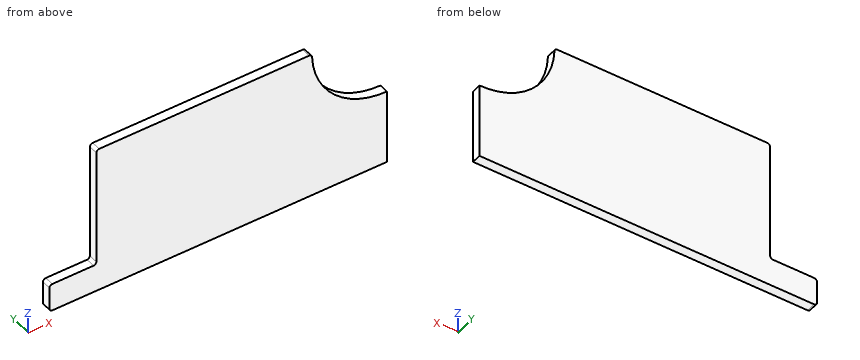
Autodesk Inventor part; units mm, degrees
ref_plane "YZ Plane" through (0, 0, 0) normal (1, 0, 0) x (0, 1, 0)
ref_plane "XZ Plane" through (0, 0, 0) normal (0, 1, 0) x (-1, 0, 0)
ref_plane "XY Plane" through (0, 0, 0) normal (0, 0, 1) x (1, 0, 0)
sketch "Esboço1" plane through (0, 0, 0) normal (0, 1, 0) x (-1, 0, 0)
  line L0 (-900, 400) -> (900, 400) construction
  line L1 (900, 400) -> (900, -400) construction
  line L2 (900, -400) -> (-900, -400) construction
  line L3 (-900, -400) -> (-900, 400) construction
  line L4 (-900, 400) -> (900, -400) construction
  line L5 (900, 400) -> (-900, -400) construction
  line L6 (900, -250) -> (650, -250) construction
  line L7 (650, -250) -> (650, 400) construction
  arc A0 (885, -400) -> (900, -385) centre (885, -385) ccw
  arc A1 (650, -235) -> (665, -250) centre (665, -235) ccw
  line L8 (885, -400) -> (-900, -400)
  line L9 (900, -385) -> (900, -250) construction
  line L10 (900, -250) -> (665, -250) construction
  line L11 (-900, -400) -> (-1700, -400) construction
  line L12 (-1700, -400) -> (-1700, 1400) construction
  line L13 (-1700, 1400) -> (-900, 1400) construction
  line L14 (-900, 1400) -> (-900, -400) construction
  circle A2 centre (-900, 400) radius 400 construction
  line L15 (900, 0) -> (-900, 0) construction
  line L16 (-1300, 1400) -> (-1300, -404.7673) construction
  arc A3 (-485.2712, 400) -> (-500.2614, 385.5422) centre (-485.2712, 385) ccw
  line L17 (650, -235) -> (650, 385)
  arc A4 (650, 385) -> (635, 400) centre (635, 385) ccw
  line L18 (635, 400) -> (-485.2712, 400)
  arc A5 (-900, 0) -> (-500.2614, 385.5422) centre (-900, 400) ccw
  line L19 (-900, -400) -> (-900, 0)
  arc A6 (900, -265) -> (885, -250) centre (885, -265) ccw
  line L20 (900, -265) -> (900, -385)
  line L21 (885, -250) -> (665, -250)
  point P0 (0, 0)
  dimension "d11" = 800
  dimension "d0" = 800
  dimension "d1" = 1800
  dimension "d3" = 650
  dimension "d5" = 15
  dimension "d6" = 800
  dimension "d7" = 1800
  dimension "d9" = 250
  dimension "d13" = 400
  dimension "d14" = 400
  dimension "d15" = 400
sketch "Esboço3" plane through (0, 0, 0) normal (0, 1, 0) x (-1, 0, 0)
  line L0 (-900, 400) -> (900, 400) construction
  line L1 (900, 400) -> (900, -400) construction
  line L2 (900, -400) -> (-900, -400) construction
  line L3 (-900, -400) -> (-900, 400) construction
  line L4 (-900, 400) -> (900, -400) construction
  line L5 (900, 400) -> (-900, -400) construction
  arc A0 (-900, -350) -> (-850, -400) centre (-850, -350) ccw
  arc A1 (850, -400) -> (900, -350) centre (850, -350) ccw
  line L6 (900, 0) -> (-900, 0) construction
  line L7 (700, 400) -> (700, 0) construction
  line L8 (850, -400) -> (-850, -400)
  line L9 (900, -350) -> (900, 400)
  line L10 (-900, -350) -> (-900, -350)
  line L11 (-900, -309.491) -> (-900, -350)
  arc A2 (-850, 400) -> (-900, 350) centre (-850, 350) ccw
  line L12 (-900, -309.491) -> (-900, 350)
  circle A3 centre (300, 400) radius 400 construction
  arc A4 (-97.5232, 355.5556) -> (-147.2136, 400) centre (-147.2136, 350) ccw
  line L13 (900, 400) -> (700, 400)
  line L14 (-147.2136, 400) -> (-850, 400)
  arc A5 (-97.5232, 355.5556) -> (700, 400) centre (300, 400) ccw
  point P0 (0, 0)
  point P1 (-498.6068, 400)
  dimension "d16" = 1800
  dimension "d17" = 800
  dimension "d19" = 200
  dimension "d20" = 50
  dimension "d21" = 800
extrude "Extrusão1" add sketch "Esboço1" along normal mid plane 50
equation "\"d6\" = d0"
equation "\"d7\" = d1"
properties part number "Lado Esquerdo Mesa"
Work out the finished part from the listing and answer in its coordinate system (mm). Give positions to 0.01 mm unless a question says otherwise; leave off trailing zeros. Order: outer loops, then holes, each group sorted by start corner. A loop starts at its lowest first (then second) coordinate and runs counter-clockwise, first axis right, second up. Notation, with made-up numbers: M 61.5,20 L 72.5,20 A26 ccw 72.5,34 Z; hole C -17,57.25 d1. An arc over 180 degrees is marked long. Return JSON: item names as keys, results as strings.
1) Section C-C, the plane x = -705 is taken. Write down the section's boundary in (y, z), plus the area to 3 significant figures.
Resolved:
{"outline": "M -25,-400 L 25,-400 L 25,-250 L -25,-250 Z", "area": "7,500 mm^2"}
2) Each of these flat-tipped pins is pushed along its axis until it touches: pin 1 (2 mm diameter, centred on y = 4, z = 311.5, fed in from -X); pin 2 (6 mm diameter, centred on y = 7, z = 231, fed in from +X). Where does it stop, or does it pass through?
Resolved:
{"pin 1": "x = -650", "pin 2": "x = 538.87"}
3) Section A-A, the plane y = -16 is taken. Write down the section's boundary in (x, z), plus the area to 3 significant figures.
Resolved:
{"outline": "M -900,-385 A15 ccw -885,-400 L 900,-400 L 900,0 A400 cw 500.26,385.54 A15 ccw 485.27,400 L -635,400 A15 ccw -650,385 L -650,-235 A15 cw -665,-250 L -885,-250 A15 ccw -900,-265 Z", "area": "1,150,000 mm^2"}
4) Straight lines are drawn through the part: line 1 along X through (y, z) = (-18, -121); line 2 along Z through (x, y) = (-786, -12); line 3 along Z through (x, y) = (616.5, 2.5). For each, find the intervals that lie inside material, in ascending order. Write a range as [from, to].
Resolved:
{"line 1": "[-650, 900]", "line 2": "[-400, -250]", "line 3": "[-400, 117.82]"}
5) Section B-B, the plane z = -116 is taken. Write down the section's boundary in (x, y), plus the area to 3 significant figures.
Resolved:
{"outline": "M -650,-25 L 900,-25 L 900,25 L -650,25 Z", "area": "77,500 mm^2"}
